CAD build for the part. Positions are in the model's coordinates, mm. A direction names the side the tool comes from. Coordinates: 2 decimals unless noted, no trailing zeros. Write each loop counter-clockwise with the first axis right and the second up, starting at its lowest first coordinate (ties: lowest second). Pieces come first, ordered by that corner, then holes. Notation, with made-up numbers: (53, 40.5) - (57, 40.5) arc R32 ccw to (57, 77.5) - close; hole circle Ø5 at (80, 21). An arc over 180 degrees is marked (long way). Answer in a Markdown table with one row per item. Add a question column.
Q1. Band-saw the part on A-A (y = 0). List the corners of the cut face in (x, z), and give its area (3 significant figures).
Q2. Drill centre lines: line 1 along Z through (x, y) = (0, 4.5); line 2 along Y through (x, z) = (0.25, -1.5); line 3 along Z through (x, y) = (-6, -8.25). Where is each one in solid material? Low to high. Write a range as from..to.
Q3. Pin check, flat tips, straight feed: pin 1 (1 mm diameter, centred on x = 4, y = 0.5, fed in from -Z); pin 2 (2 mm diameter, centred on y = -1.5, z = -5, fed in from -X); pin 3 (5 mm diameter, centred on x = -5, z = -14.5, fed in from +Y). Stop position of each tip, or through.
Q4. 3-axis set-ups, long thin cutter, end or side, ignore diameter. For faces 1 (the cylindrical face through (0, -1, 3)), 2 (the flat face through (0, 0, -35.3)), 3 (the cylindrical face through (-2.038, -9.176, -24.983)): which of +Z, -Z, +X, -X, +Y, -Y reach the whole face in a straight line?
Q5. Band-saw the part on C-C (z = -9). List the corners of the cut face in (x, y), and give its area (3 significant figures).
```python
from build123d import *

# Parameters (mm, degrees)
SKETCH1_R                = 11.75
SKETCH1_R_2              = 9.4
BOSS_EXTRUDE1_DEPTH      = 23.8
SKETCH1_3_R              = 9.4
SKETCH1_3_R_2            = 4.25
BOSS_EXTRUDE2_DEPTH      = 27.2
SKETCH1_4_R              = 4.25
SKETCH1_4_R_2            = 2.85
BOSS_EXTRUDE3_DEPTH      = 29.4
SKETCH1_5_R              = 2.85
BOSS_EXTRUDE4_DEPTH      = 2.3
BOSS_EXTRUDE4_DEPTH_BACK = 29.4
SKETCH1_6_R              = 1
BOSS_EXTRUDE5_DEPTH      = 3.3
BOSS_EXTRUDE5_DEPTH_BACK = 35.3
FILLET1_R                = 1


with BuildPart() as part:
    # Sketch1 → Boss-Extrude1 (new body)
    with BuildSketch(Plane.XY):
        Circle(SKETCH1_R)
        Circle(SKETCH1_R_2, mode=Mode.SUBTRACT)
    extrude(amount=-BOSS_EXTRUDE1_DEPTH)

    # Sketch1_3 → Boss-Extrude2 (add)
    with BuildSketch(Plane.XY):
        Circle(SKETCH1_3_R)
        Circle(SKETCH1_3_R_2, mode=Mode.SUBTRACT)
    extrude(amount=-BOSS_EXTRUDE2_DEPTH)

    # Sketch1_4 → Boss-Extrude3 (add)
    with BuildSketch(Plane.XY):
        Circle(SKETCH1_4_R)
        Circle(SKETCH1_4_R_2, mode=Mode.SUBTRACT)
    extrude(amount=-BOSS_EXTRUDE3_DEPTH)

    # Sketch1_5 → Boss-Extrude4 (add, two sides)
    with BuildSketch(Plane.XY) as boss_extrude4_sk:
        Circle(SKETCH1_5_R)
    extrude(amount=BOSS_EXTRUDE4_DEPTH)
    extrude(boss_extrude4_sk.sketch, amount=-BOSS_EXTRUDE4_DEPTH_BACK)

    # Sketch1_6 → Boss-Extrude5 (add, two sides)
    with BuildSketch(Plane.XY) as boss_extrude5_sk:
        Circle(SKETCH1_6_R)
    extrude(amount=BOSS_EXTRUDE5_DEPTH)
    extrude(boss_extrude5_sk.sketch, amount=-BOSS_EXTRUDE5_DEPTH_BACK)

    # Fillet1
    fillet1_edges = [part.edges().sort_by_distance(p)[0] for p in [
        (-11.75, 0, -23.8),
        (-9.4, 0, -27.2),
    ]]
    fillet(fillet1_edges, radius=FILLET1_R)


solid = part.part
```
Checked values:
| question | item | result |
|---|---|---|
| 1 | outline | (-11.75, -22.8) arc R1 ccw to (-10.75, -23.8) - (-9.4, -23.8) - (-9.4, -26.2) arc R1 ccw to (-8.4, -27.2) - (-4.25, -27.2) - (-4.25, -29.4) - (-1, -29.4) - (-1, -35.3) - (1, -35.3) - (1, -29.4) - (4.25, -29.4) - (4.25, -27.2) - (8.4, -27.2) arc R1 ccw to (9.4, -26.2) - (9.4, -23.8) - (10.75, -23.8) arc R1 ccw to (11.75, -22.8) - (11.75, 0) - (2.85, 0) - (2.85, 2.3) - (1, 2.3) - (1, 3.3) - (-1, 3.3) - (-1, 2.3) - (-2.85, 2.3) - (-2.85, 0) - (-11.75, 0) - close |
| 1 | area | 668 mm² |
| 2 | line 1 | z = -27.2..0 |
| 2 | line 2 | y = -11.75..11.75 |
| 2 | line 3 | z = -23.8..0 |
| 3 | pin 1 | stops at z = -29.4 |
| 3 | pin 2 | stops at x = -11.74 |
| 3 | pin 3 | stops at y = 11.48 |
| 4 | face 1 | +Z |
| 4 | face 2 | -Z, +X, -X, +Y, -Y |
| 4 | face 3 | -Z |
| 5 | outline | circle Ø23.5 at (0, 0) |
| 5 | area | 434 mm² |
